Work out the finished part from the listing and answer in its coordinate system (mm). Face numbers are marked on the shaded views. Round coordinates to 2 decimals unless told otherwise and drop trailing zeros. Order: outer loops, then holes, each group sorted by start corner. A loop starts at its lowest first (then second) coordinate and runs counter-clockwise, first axis right, second up. Notation, with made-up numbers: M 14,5.25 L 38,5.25 A18 ccw 38,39.25 Z; hole C 81.5,-2.5 d10. An arc over 180 degrees is marked long. Answer as a JSON object with one key per item and string values. Group by question number.
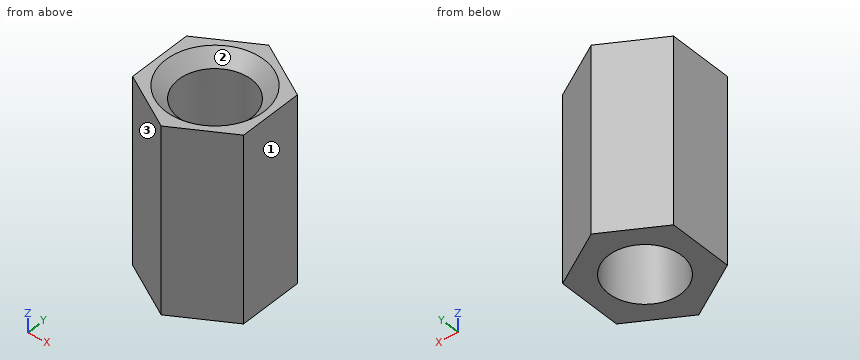
Autodesk Inventor part; units mm, degrees
ref_plane "YZ Plane" through (0, 0, 0) normal (1, 0, 0) x (0, 1, 0)
ref_plane "XZ Plane" through (0, 0, 0) normal (0, 1, 0) x (-1, 0, 0)
ref_plane "XY Plane" through (0, 0, 0) normal (0, 0, 1) x (1, 0, 0)
sketch "Sketch1" plane through (0, 0, 0) normal (0, 0, 1) x (1, 0, 0)
  line L0 (0, 12.7583) -> (11.049, 6.3791)
  line L1 (11.049, 6.3791) -> (11.049, -6.3791)
  line L2 (11.049, -6.3791) -> (0, -12.7583)
  line L3 (0, -12.7583) -> (-11.049, -6.3791)
  line L4 (-11.049, -6.3791) -> (-11.049, 6.3791)
  line L5 (-11.049, 6.3791) -> (0, 12.7583)
  point P0 (0, 0)
  point P1 (0, 0)
  dimension "d0" = 22.098
extrude "Extrusion1" add sketch "Sketch1" along normal blind 37.084
sketch "Sketch2" plane through (0, 0, 37.084) normal (0, 0, 1) x (1, 0, 0)
  circle A0 centre (0, 0) radius 7.239
  dimension "d4" = 14.478
extrude "Extrusion2" cut sketch "Sketch2" against normal blind 37.084
chamfer "Chamfer1" distance 2.54 angle 45 1 edges at (-7.239, 0, 37.084)
thread "Thread1"
thread "Thread2"
properties part number "inside thread"
Item 1: Each of these flat-tipped pins is pushed along its axis until it touches: pin 1 (10 mm diameter, centred on y = 10, z = 31.5, fed in from +X); pin 2 (8 mm diameter, centred on x = 3.5, z = 7.5, fed in from +Y); pin 3 (3 mm diameter, centred on x = -6, z = 10, fed in from +Y); pin 4 (12 mm diameter, centred on x = 3, y = 1.5, fed in from +Z). Where does it stop, or does it pass through?
Item 2: Consider L1, parallel to Y at x = 0, z = 23.5; L2, parallel to X at y = 0.25, z = 28; L3, parallel to X at y = 5.75, z = 24.5. Determine where each line is inside the solid, lowest interval first.
Item 3: Find section B-B (y = 0). Give the vertices of the cut face in (x, z).
Item 4: The mould has two halves that part along X. Classify the marked faces 1, 2 and 3: +X half, -X half, draft (parallel to the pull), parting line (faces both ways), or undercut.
Item 5: Find section A-A (z = 14). Give the vertices of the cut face in (x, y), and give its area (3 significant figures).
Responses:
{
 "1": {"pin 1": "stops at x = 11.05", "pin 2": "stops at y = 12.76", "pin 3": "stops at y = 10.16", "pin 4": "stops at z = 36.66"},
 "2": {"L1": "y = -12.76 to -7.24, 7.24 to 12.76", "L2": "x = -11.05 to -7.23, 7.23 to 11.05", "L3": "x = -11.05 to -4.4, 4.4 to 11.05"},
 "3": {"outline": "M -11.05,0 L -7.24,0 L -7.24,34.54 L -9.78,37.08 L -11.05,37.08 Z; M 7.24,0 L 11.05,0 L 11.05,37.08 L 9.78,37.08 L 7.24,34.54 Z"},
 "4": {"face 1": "+X half", "face 2": "undercut", "face 3": "-X half"},
 "5": {"outline": "M -11.05,-6.38 L 0,-12.76 L 11.05,-6.38 L 11.05,6.38 L 0,12.76 L -11.05,6.38 Z; hole C 0,0 d14.48", "area": "258 mm^2"}
}
